from build123d import *

# Parameters (mm, degrees)
F0_R      = 19.75
F0_R_2    = 15.5
F1_DEPTH  = 28
F2_DEPTH  = 8
F4_DEPTH  = 50
F7_R      = 20
F8_DEPTH  = 0.5
F10_R     = 20
F11_DEPTH = 0.5
F13_R     = 20
F14_DEPTH = 0.5
F16_DEPTH = 50


with BuildPart() as f1:
    # F0 (on Top) → F1 (new body)
    with BuildSketch(Plane.XY):
        Circle(F0_R)
        Circle(F0_R_2, mode=Mode.SUBTRACT)
    extrude(amount=F1_DEPTH)

    # F0 (on Top) → F2 (join)
    with BuildSketch(Plane.XY):
        Circle(F0_R_2)
    extrude(amount=F2_DEPTH)

    # F3 (on Front) → F4 (cut, symmetric)
    with BuildSketch(Plane.XZ):
        with BuildLine():
            ThreePointArc((0, 25), (-4, 21), (0, 17))
            Line((0, 17), (0, 21))
            Line((0, 21), (0, 25))
        make_face()
        with BuildLine():
            Line((0, 21), (0, 17))
            ThreePointArc((0, 17), (2.828427, 18.171573), (4, 21))
            ThreePointArc((4, 21), (2.828427, 23.828427), (0, 25))
            Line((0, 25), (0, 21))
        make_face()
    extrude(amount=F4_DEPTH, both=True, mode=Mode.SUBTRACT)

    # F7 (on plane+point) → F8 (join, symmetric)
    with BuildSketch(Plane.XY.offset(4)):
        Circle(F7_R)
    extrude(amount=F8_DEPTH, both=True)

    # F10 (on plane+point) → F11 (join, symmetric)
    with BuildSketch(Plane.XY.offset(8)):
        Circle(F10_R)
    extrude(amount=F11_DEPTH, both=True)

    # F13 (on plane+point) → F14 (join, symmetric)
    with BuildSketch(Plane.XY.offset(12)):
        Circle(F13_R)
    extrude(amount=F14_DEPTH, both=True)

    # F15 (on Right) → F16 (cut, symmetric)
    with BuildSketch(Plane.YZ):
        with BuildLine():
            ThreePointArc((-14, 28), (-9.899495, 18.100505), (0, 14))
            Line((0, 14), (0, 28))
            Line((0, 28), (-14, 28))
        make_face()
        with BuildLine():
            Line((0, 28), (0, 14))
            ThreePointArc((0, 14), (9.899495, 18.100505), (14, 28))
            Line((14, 28), (0, 28))
        make_face()
    extrude(amount=F16_DEPTH, both=True, mode=Mode.SUBTRACT)


solid = f1.part
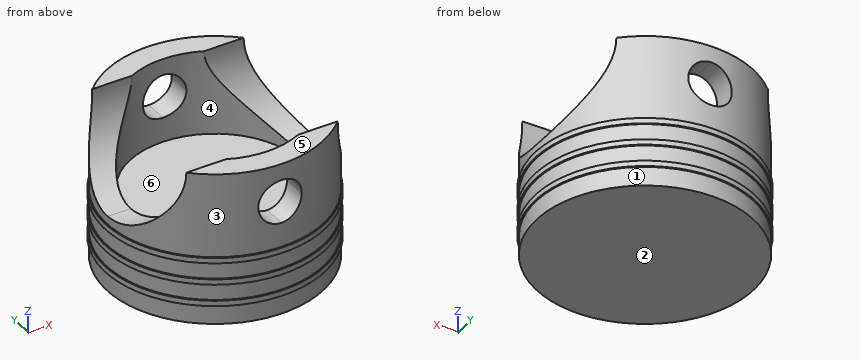
Check sheet for the modelled part. Datum: model origin and axes. Units: mm. Face numbers are marked on the shaded views. A direction names the side the tool comes from. Round coordinates to 2 decimals unless told otherwise and drop trailing zeros. Write each loop counter-clockwise with the first axis right and the second up, starting at its lowest first coordinate (ties: lowest second). Pieces come first, ordered by that corner, then holes. Notation, with made-up numbers: (-11, -19.75) -> (45, -19.75) arc R10 cw to (45, -9.75) -> close; hole circle Ø6 at (-12.5, 80). An arc over 180 degrees is marked (long way). Answer as CSV lines item,"result". Start each with the question number.
1) Section check B-B on x = 2. State how many separate pieces and enclosed holes the cut face has, and give its area (3 significant figures).
2) Tool access check on the marked faces 1 and 2. Record the directions out of +Z, -Z, +X, -X, +Y, -Y that give a thin tool (end or side, any length) a straight path to the whole face; none if there is none.
3) Section check A-A on z = 18.5. Enter the section's corners in (x, y).
4) Material ranges on line 1 (Z direction, x = 8, y = -6); line 2 (Y direction, x = 0, z = 10.6); line 3 (Z direction, x = -15, y = -13), recorded low to high. Write a range as from..to.
5) Go/stop test with flat-tipped pins: P1, Ø2, axis at x = -13.5, z = 12, coming from the -Y side; P2, Ø2, axis at x = -7.5, y = -8.5, coming from the +Z side; P3, Ø2, axis at y = -2.5, z = 3.5, coming from the -X side; P4, Ø12, axis at x = -0.5, y = 2.5, coming from the -Z side. Record where each tip stops, or that it passes through.
6) Release check for a two-part mould opening along Y. For the marked faces 3, 4, 5 and 6 record: pulls with the +Y half, pulls with the -Y half, needs draft (parallel to the pull), parting line crosses it, or undercut.
7) Section check D-D on z = 5.75. Enter the section's corners in (x, y).
8) Section check C-C on x = 17. Enter the section's corners in (y, z), and give its area (3 significant figures).
Found:
1,separate pieces,"3"
1,enclosed holes,"1"
1,area,"474 mm^2"
2,face 1,"-Z"
2,face 2,"-Z, +X, -X, +Y, -Y"
3,outline,"(-16.86, -10.28) arc R19.75 ccw to (-3.12, -19.5) -> (-3.12, -15.18) arc R15.5 cw to (-11.6, -10.28) -> close; (-16.86, 10.28) -> (-11.6, 10.28) arc R15.5 cw to (-3.12, 15.18) -> (-3.12, 19.5) arc R19.75 ccw to start; (3.12, -19.5) arc R19.75 ccw to (16.86, -10.28) -> (11.6, -10.28) arc R15.5 cw to (3.12, -15.18) -> close; (3.12, 15.18) arc R15.5 cw to (11.6, 10.28) -> (16.86, 10.28) arc R19.75 ccw to (3.12, 19.5) -> close"
4,line 1,"z = 0..8.5, 11.5..12.5"
4,line 2,"y = -19.75..-15.5, 15.5..19.75"
4,line 3,"z = 3.5..4.5, 7.5..8.5, 11.5..12.5"
5,P1,"stops at y = -15.61"
5,P2,"stops at z = 12.5"
5,P3,"stops at x = -19.94"
5,P4,"stops at z = 0"
6,face 3,"parting line crosses it"
6,face 4,"undercut"
6,face 5,"needs draft"
6,face 6,"undercut"
7,outline,"circle Ø39.5 at (0, 0)"
8,outline,"(-10.54, 3.5) -> (-10.05, 3.5) -> (-10.05, 0) -> (10.05, 0) -> (10.05, 3.5) -> (10.54, 3.5) -> (10.54, 4.5) -> (10.05, 4.5) -> (10.05, 7.5) -> (10.54, 7.5) -> (10.54, 8.5) -> (10.05, 8.5) -> (10.05, 11.5) -> (10.54, 11.5) -> (10.54, 12.5) -> (10.05, 12.5) -> (10.05, 18.26) arc R14 cw to (-10.05, 18.26) -> (-10.05, 12.5) -> (-10.54, 12.5) -> (-10.54, 11.5) -> (-10.05, 11.5) -> (-10.05, 8.5) -> (-10.54, 8.5) -> (-10.54, 7.5) -> (-10.05, 7.5) -> (-10.05, 4.5) -> (-10.54, 4.5) -> close"
8,area,"311 mm^2"
